Part model, mm, in its own coordinate system. A direction names the side the tool comes from. Give positions to 0.01 mm unless a question says otherwise; leave off trailing zeros. Write each loop counter-clockwise with the first axis right and the second up, starting at its lowest first coordinate (ties: lowest second). Pieces come first, ordered by that corner, then holes. Notation, with made-up numbers: M 3,-30 L 32,-30 A24 ccw 32,-19 Z; hole C -25.5,18 d3. An arc over 180 degrees is marked long. Answer as CSV lines item,"result". Start each with the question number.
1) Slice it at D-D, the plane y = 70. Give the cut face in (x, z).
2) Mould opens along X. For faces 4 (the cylindrical face through (-0.5, 253.35, -9.92)), 5 (the flat face through (33.756, 249, 40)), 6 (the flat face through (1, 38.1, 1)) say: pulls with the +X half, pulls with the -X half, needs draft (parallel to the pull), parting line crosses it, or undercut.
3) Slice it at B-B, the plane x = 71.5. Give the cut face in (y, z).
4) Slice it at A-A, the plane y = 177.8. Give the cut face in (x, z) (3 decimals), plus the area to 3 significant figures.
5) Pin check, flat tips, straight feed: pin 1 Ø4 at (y, z) = (184, -81) entering from -X; pin 2 Ø5 at (x, y) = (25.5, 195) entering from -Z (3 decimals); pin 3 Ø1 at (y, z) = (43.5, -52.5) entering from -X. Stop position of each tip, or through.
6) Wall check: line 1 along X through (y, z) = (13, 0); line 2 along Y through (x, z) = (-20, 0); line 3 along Y through (x, z) = (86.5, -40.5). Give the ranges that are in metal, low to high. Write a range as from..to.
7) Tool access for faces 1 (the flat face through (-33.808, 249, 40)), 2 (the flat face through (-1, 76.2, -109)), 3 (the flat face through (0, 170, 93.345)): list every direction of +Z, -Z, +X, -X, +Y, -Y with a clear straight run to the whole face (end or side of a thin tool).
8) Slice it at C-C, the plane y = 108. Give the cut face in (x, z) (3 decimals), plus the area to 3 significant figures.
```python
from build123d import *

# Parameters (mm, degrees)
SKETCH1_R           = 114.3
BOSS_EXTRUDE1_DEPTH = 76.2
SKETCH3_W           = 67.564
SKETCH3_H           = 186.69
BOSS_EXTRUDE3_DEPTH = 203.2
SKETCH4_R           = 76.2
CUT_EXTRUDE1_DEPTH  = 127
FILLET1_SIZE        = 25.4
FILLET2_SIZE        = 12.7
SKETCH2_R           = 88.9
CUT_EXTRUDE2_DEPTH  = 38.1


with BuildPart() as part:
    # Sketch1 → Boss-Extrude1 (new body)
    with BuildSketch(Plane(origin=(0, 0, 0), x_dir=(1, 0, 0), z_dir=(0, 1, 0))):
        with Locations(Location((0, 0, 0), (0, 0, 90))):
            Circle(SKETCH1_R)
    extrude(amount=BOSS_EXTRUDE1_DEPTH)

    # Sketch3 → Boss-Extrude3 (add)
    with BuildSketch(Plane(origin=(0, 76.2, 0), x_dir=(1, 0, 0), z_dir=(0, 1, 0))):
        with Locations((-0.02614759, 0)):
            Rectangle(SKETCH3_W, SKETCH3_H)
    extrude(amount=BOSS_EXTRUDE3_DEPTH)

    # Sketch4 → Cut-Extrude1 (cut)
    with BuildSketch(Plane.ZY.offset(33.80814759)):
        with Locations((0, 177.8)):
            Circle(SKETCH4_R)
    extrude(amount=-CUT_EXTRUDE1_DEPTH, mode=Mode.SUBTRACT)

    # Fillet1
    # a fillet whose section is not a circle: 25.4 mm, written as the material it takes off along each edge
    with BuildSketch(Plane(origin=(97.25585241, 279.4, 93.345), x_dir=(0, -1, 0), z_dir=(-1, 0, 0)), Plane(origin=(-97.30814759, 279.4, -93.345), x_dir=(0, -1, 0), z_dir=(1, 0, 0))) as fillet1_piece_1:
        with BuildLine():
            Bezier((FILLET1_SIZE, 0), (0, 0), (0, -FILLET1_SIZE), weights=[1, 1, 1])
            Line((0, -FILLET1_SIZE), (0, 0))
            Line((0, 0), (FILLET1_SIZE, 0))
        make_face()
    extrude(amount=194.564, mode=Mode.SUBTRACT)

    # Fillet2
    # a fillet whose section is not a circle: 12.7 mm, written as the material it adds along each edge
    with BuildSketch(Plane(origin=(33.75585241, 76.2, 93.345), x_dir=(0, 0, 1), z_dir=(-1, 0, 0)), Plane(origin=(-33.80814759, 76.2, -93.345), x_dir=(0, 0, -1), z_dir=(1, 0, 0))) as fillet2_piece_1:
        with BuildLine():
            Bezier((FILLET2_SIZE, 0), (0, 0), (0, FILLET2_SIZE), weights=[1, 1, 1])
            Line((0, FILLET2_SIZE), (0, 0))
            Line((0, 0), (FILLET2_SIZE, 0))
        make_face()
    extrude(amount=67.564)
    with BuildSketch(Plane(origin=(-33.80814759, 76.2, 93.345), x_dir=(-1, 0, 0), z_dir=(0, 0, -1)), Plane(origin=(33.75585241, 76.2, -93.345), x_dir=(1, 0, 0), z_dir=(0, 0, 1))) as fillet2_piece_2:
        with BuildLine():
            Bezier((FILLET2_SIZE, 0), (0, 0), (0, FILLET2_SIZE), weights=[1, 1, 1])
            Line((0, FILLET2_SIZE), (0, 0))
            Line((0, 0), (FILLET2_SIZE, 0))
        make_face()
    extrude(amount=186.69)
    with BuildSketch(Plane(origin=(65.50585241, 76.2, 93.345), x_dir=(0, 0, 1), z_dir=(-1, 0, 0))) as fillet2_piece_3a_section:
        with BuildLine():
            Bezier((FILLET2_SIZE, 0), (0, 0), (0, FILLET2_SIZE), weights=[1, 1, 1])
            Line((0, FILLET2_SIZE), (0, 0))
            Line((0, 0), (FILLET2_SIZE, 0))
        make_face()
    fillet2_piece_3a = extrude(amount=99.314, mode=Mode.PRIVATE)
    fillet2_piece_3a = fillet2_piece_3a & Plane(origin=(0, 76.2, 0), x_dir=(0, 0, -1), z_dir=(0, -1, 0)) * Cylinder(114.3, 250, mode=Mode.PRIVATE)
    fillet2_piece_3a = split(fillet2_piece_3a, bisect_by=Plane(origin=(33.75585241, 76.2, 93.345), z_dir=(1, 0, 0)), keep=Keep.TOP, mode=Mode.PRIVATE)
    with BuildSketch(Plane(origin=(33.75585241, 76.2, -93.345), x_dir=(1, 0, 0), z_dir=(0, 0, 1))) as fillet2_piece_3b_section:
        with BuildLine():
            Bezier((FILLET2_SIZE, 0), (0, 0), (0, FILLET2_SIZE), weights=[1, 1, 1])
            Line((0, FILLET2_SIZE), (0, 0))
            Line((0, 0), (FILLET2_SIZE, 0))
        make_face()
    fillet2_piece_3b = extrude(amount=218.44, mode=Mode.PRIVATE)
    fillet2_piece_3b = fillet2_piece_3b & Plane(origin=(0, 76.2, 0), x_dir=(0, 0, -1), z_dir=(0, -1, 0)) * Cylinder(114.3, 488, mode=Mode.PRIVATE)
    fillet2_piece_3b = split(fillet2_piece_3b, bisect_by=Plane(origin=(33.75585241, 76.2, 93.345), z_dir=(0, 0, 1)), keep=Keep.TOP, mode=Mode.PRIVATE)
    fillet2_piece_3 = fillet2_piece_3a & fillet2_piece_3b
    add(fillet2_piece_3)
    with BuildSketch(Plane(origin=(-33.80814759, 76.2, 125.095), x_dir=(-1, 0, 0), z_dir=(0, 0, -1))) as fillet2_piece_4a_section:
        with BuildLine():
            Bezier((FILLET2_SIZE, 0), (0, 0), (0, FILLET2_SIZE), weights=[1, 1, 1])
            Line((0, FILLET2_SIZE), (0, 0))
            Line((0, 0), (FILLET2_SIZE, 0))
        make_face()
    fillet2_piece_4a = extrude(amount=218.44, mode=Mode.PRIVATE)
    fillet2_piece_4a = fillet2_piece_4a & Plane(origin=(0, 76.2, 0), x_dir=(0, 0, -1), z_dir=(0, -1, 0)) * Cylinder(114.3, 488, mode=Mode.PRIVATE)
    fillet2_piece_4a = split(fillet2_piece_4a, bisect_by=Plane(origin=(-33.80814759, 76.2, 93.345), z_dir=(0, 0, 1)), keep=Keep.TOP, mode=Mode.PRIVATE)
    with BuildSketch(Plane(origin=(33.75585241, 76.2, 93.345), x_dir=(0, 0, 1), z_dir=(-1, 0, 0))) as fillet2_piece_4b_section:
        with BuildLine():
            Bezier((FILLET2_SIZE, 0), (0, 0), (0, FILLET2_SIZE), weights=[1, 1, 1])
            Line((0, FILLET2_SIZE), (0, 0))
            Line((0, 0), (FILLET2_SIZE, 0))
        make_face()
    fillet2_piece_4b = extrude(amount=99.314, mode=Mode.PRIVATE)
    fillet2_piece_4b = fillet2_piece_4b & Plane(origin=(0, 76.2, 0), x_dir=(0, 0, -1), z_dir=(0, -1, 0)) * Cylinder(114.3, 250, mode=Mode.PRIVATE)
    fillet2_piece_4b = split(fillet2_piece_4b, bisect_by=Plane(origin=(-33.80814759, 76.2, 93.345), z_dir=(-1, 0, 0)), keep=Keep.TOP, mode=Mode.PRIVATE)
    fillet2_piece_4 = fillet2_piece_4a & fillet2_piece_4b
    add(fillet2_piece_4)
    with BuildSketch(Plane(origin=(-33.80814759, 76.2, 93.345), x_dir=(-1, 0, 0), z_dir=(0, 0, -1))) as fillet2_piece_5a_section:
        with BuildLine():
            Bezier((FILLET2_SIZE, 0), (0, 0), (0, FILLET2_SIZE), weights=[1, 1, 1])
            Line((0, FILLET2_SIZE), (0, 0))
            Line((0, 0), (FILLET2_SIZE, 0))
        make_face()
    fillet2_piece_5a = extrude(amount=218.44, mode=Mode.PRIVATE)
    fillet2_piece_5a = fillet2_piece_5a & Plane(origin=(0, 76.2, 0), x_dir=(0, 0, -1), z_dir=(0, -1, 0)) * Cylinder(114.3, 488, mode=Mode.PRIVATE)
    fillet2_piece_5a = split(fillet2_piece_5a, bisect_by=Plane(origin=(-33.80814759, 76.2, -93.345), z_dir=(0, 0, -1)), keep=Keep.TOP, mode=Mode.PRIVATE)
    with BuildSketch(Plane(origin=(-65.55814759, 76.2, -93.345), x_dir=(0, 0, -1), z_dir=(1, 0, 0))) as fillet2_piece_5b_section:
        with BuildLine():
            Bezier((FILLET2_SIZE, 0), (0, 0), (0, FILLET2_SIZE), weights=[1, 1, 1])
            Line((0, FILLET2_SIZE), (0, 0))
            Line((0, 0), (FILLET2_SIZE, 0))
        make_face()
    fillet2_piece_5b = extrude(amount=99.314, mode=Mode.PRIVATE)
    fillet2_piece_5b = fillet2_piece_5b & Plane(origin=(0, 76.2, 0), x_dir=(0, 0, -1), z_dir=(0, -1, 0)) * Cylinder(114.3, 250, mode=Mode.PRIVATE)
    fillet2_piece_5b = split(fillet2_piece_5b, bisect_by=Plane(origin=(-33.80814759, 76.2, -93.345), z_dir=(-1, 0, 0)), keep=Keep.TOP, mode=Mode.PRIVATE)
    fillet2_piece_5 = fillet2_piece_5a & fillet2_piece_5b
    add(fillet2_piece_5)
    with BuildSketch(Plane(origin=(33.75585241, 76.2, -125.095), x_dir=(1, 0, 0), z_dir=(0, 0, 1))) as fillet2_piece_6a_section:
        with BuildLine():
            Bezier((FILLET2_SIZE, 0), (0, 0), (0, FILLET2_SIZE), weights=[1, 1, 1])
            Line((0, FILLET2_SIZE), (0, 0))
            Line((0, 0), (FILLET2_SIZE, 0))
        make_face()
    fillet2_piece_6a = extrude(amount=218.44, mode=Mode.PRIVATE)
    fillet2_piece_6a = fillet2_piece_6a & Plane(origin=(0, 76.2, 0), x_dir=(0, 0, -1), z_dir=(0, -1, 0)) * Cylinder(114.3, 488, mode=Mode.PRIVATE)
    fillet2_piece_6a = split(fillet2_piece_6a, bisect_by=Plane(origin=(33.75585241, 76.2, -93.345), z_dir=(0, 0, -1)), keep=Keep.TOP, mode=Mode.PRIVATE)
    with BuildSketch(Plane(origin=(-33.80814759, 76.2, -93.345), x_dir=(0, 0, -1), z_dir=(1, 0, 0))) as fillet2_piece_6b_section:
        with BuildLine():
            Bezier((FILLET2_SIZE, 0), (0, 0), (0, FILLET2_SIZE), weights=[1, 1, 1])
            Line((0, FILLET2_SIZE), (0, 0))
            Line((0, 0), (FILLET2_SIZE, 0))
        make_face()
    fillet2_piece_6b = extrude(amount=99.314, mode=Mode.PRIVATE)
    fillet2_piece_6b = fillet2_piece_6b & Plane(origin=(0, 76.2, 0), x_dir=(0, 0, -1), z_dir=(0, -1, 0)) * Cylinder(114.3, 250, mode=Mode.PRIVATE)
    fillet2_piece_6b = split(fillet2_piece_6b, bisect_by=Plane(origin=(33.75585241, 76.2, -93.345), z_dir=(1, 0, 0)), keep=Keep.TOP, mode=Mode.PRIVATE)
    fillet2_piece_6 = fillet2_piece_6a & fillet2_piece_6b
    add(fillet2_piece_6)

    # Sketch2 → Cut-Extrude2 (cut)
    with BuildSketch(Plane(origin=(0, 0, 0), x_dir=(-1, 0, 0), z_dir=(0, -1, 0))):
        with Locations(Location((0, 0, 0), (0, 0, 90))):
            Circle(SKETCH2_R)
    extrude(amount=-CUT_EXTRUDE2_DEPTH, mode=Mode.SUBTRACT)


solid = part.part
```
Found:
1,outline,"C 0,0 d228.6"
2,face 4,"needs draft"
2,face 5,"pulls with the +X half"
2,face 6,"undercut"
3,outline,"M 0,-89.18 L 76.2,-89.18 L 76.2,89.18 L 0,89.18 L 0,52.83 L 38.1,52.83 L 38.1,-52.83 L 0,-52.83 Z"
4,outline,"M -33.808,-93.345 L 33.756,-93.345 L 33.756,-76.2 L -33.808,-76.2 Z; M -33.808,76.2 L 33.756,76.2 L 33.756,93.345 L -33.808,93.345 Z"
4,area,"2,320 mm²"
5,pin 1,"x = -33.81"
5,pin 2,"z = -93.345"
5,pin 3,"x = -101.79"
6,line 1,"-114.3..-88.9, 88.9..114.3"
6,line 2,"38.1..101.6, 254..279.4"
6,line 3,"0..76.2"
7,face 1,"+Z, -Z, -X, +Y"
7,face 2,"-Z, +X, -X, +Y"
7,face 3,"+Z, +X, -X, +Y"
8,outline,"M -33.808,-93.345 L 33.756,-93.345 L 33.756,-30.568 L -33.808,-30.568 Z; M -33.808,30.568 L 33.756,30.568 L 33.756,93.345 L -33.808,93.345 Z"
8,area,"8,480 mm²"
